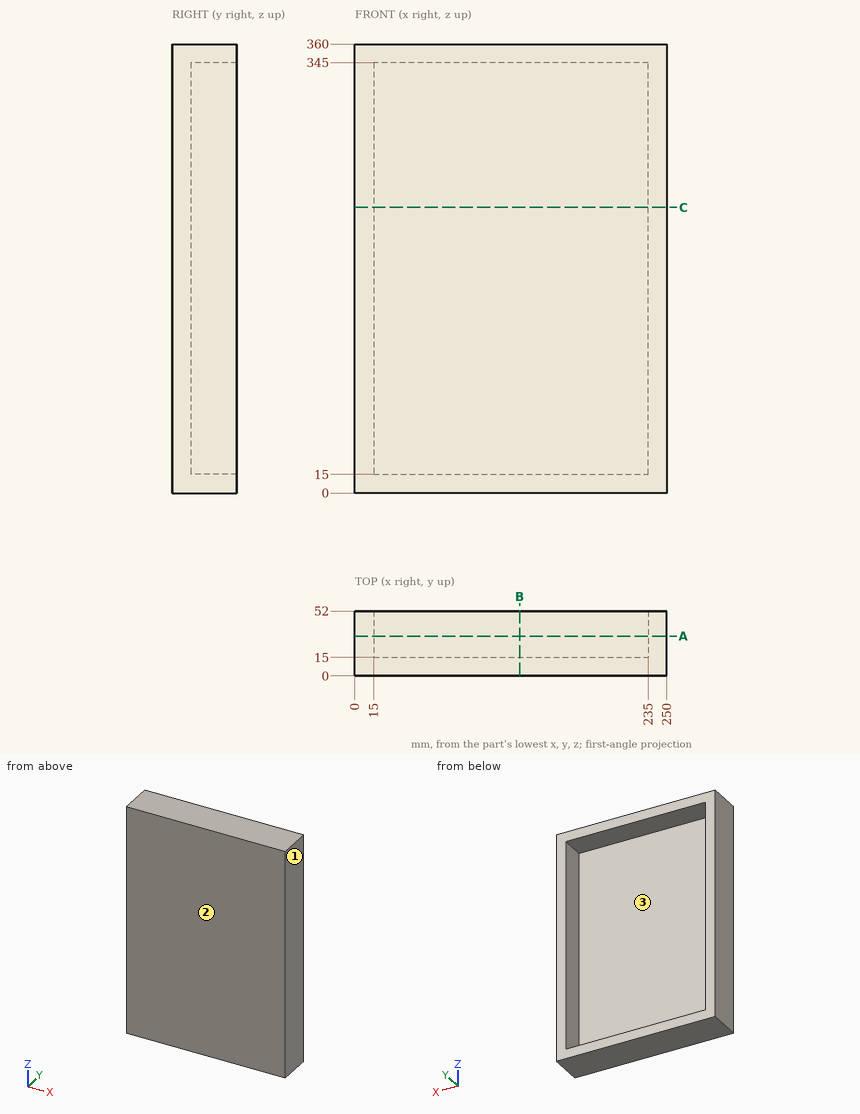
For this review, use the dimensioned drawing (mm, ordinates from the lowest corner) and the shaded views. Round coordinates to 2 decimals unless told otherwise and drop trailing zeros. Write each loop counter-clockwise with the first axis right and the second up, starting at its lowest first coordinate (ties: lowest second). Pieces come first, ordered by that corner, then holes. Notation, with made-up numbers: (22, -13.5) - (30, -13.5) arc R30 ccw to (30, 19.5) - close; hole circle Ø5 at (-17.75, 72.25). An arc over 180 degrees is marked (long way). One line per item, written item: value. Start each with the question number.
1. Consider section B-B on x = 132. Write out the cut boundary in (y, z), and give its area (3 significant figures).
2. To check wall thickness, follow L1, parallel to X at y = 18, z = 126.5; L2, parallel to Z at x = 202, y = 34.5; L3, parallel to Y at x = 66, z = 88.5. State the ranges of each line that lie inside material, in increasing order. Write a range as from..to.
3. Consider section A-A on y = 32. Write out the cut boundary in (x, z), and give its area (3 significant figures).
4. Clearance check with a flat-ended pin moving along its axis: P1, Ø1, axis at x = 186, z = 129, coming from the +Y side. State where the tip first meets the part, or that it passes through.
5. The part is to be moulded in two halves that separate along X. For the marked faces 1, 2 and 3, say which applies: released by +X, released by -X, zero draft, split by the parting line, or undercut.
6. Consider section C-C on z = 229. Write out the cut boundary in (x, y).
Checks:
1. outline: (0, 0) - (52, 0) - (52, 15) - (15, 15) - (15, 345) - (52, 345) - (52, 360) - (0, 360) - close
1. area: 6,510 mm^2
2. L1: x = 0..15, 235..250
2. L2: z = 0..15, 345..360
2. L3: y = 0..15
3. outline: (0, 0) - (250, 0) - (250, 360) - (0, 360) - close; hole (15, 15) - (235, 15) - (235, 345) - (15, 345) - close
3. area: 17,400 mm^2
4. P1: stops at y = 15
5. face 1: released by +X
5. face 2: zero draft
5. face 3: undercut
6. outline: (0, 0) - (250, 0) - (250, 52) - (235, 52) - (235, 15) - (15, 15) - (15, 52) - (0, 52) - close
